from build123d import *

# Parameters (mm, degrees)
SKIZZE1_W                       = 660
SKIZZE1_H                       = 370
AUFSATZ_LINEAR_AUSTRAGEN1_DEPTH = 200
SKIZZE2_R                       = 30
SCHNITT_LINEAR_AUSTRAGEN1_DEPTH = 566.799856976
VERRUNDUNG1_R                   = 30
SKIZZE3_W                       = 300
SKIZZE3_H                       = 270
SCHNITT_LINEAR_AUSTRAGEN2_DEPTH = 30
VERRUNDUNG2_R                   = 30
SKIZZE5_W                       = 50
SKIZZE5_H                       = 100
AUFSATZ_LINEAR_AUSTRAGEN2_DEPTH = 200


with BuildPart() as part:
    # Skizze1 → Aufsatz-Linear austragen1 (new body)
    with BuildSketch(Plane.XY):
        with Locations((-48.456705786, -9.625748503)):
            Rectangle(SKIZZE1_W, SKIZZE1_H)
    extrude(amount=AUFSATZ_LINEAR_AUSTRAGEN1_DEPTH)

    # Skizze2 → Schnitt-Linear austragen1 (cut, through all)
    with BuildSketch(Plane.XZ.offset(194.625748503)):
        with Locations(Location((-303.456705786, 80, 0), (0, 0, 270))):
            Circle(SKIZZE2_R)
        with Locations(Location((206.543294214, 80, 0), (0, 0, 270))):
            Circle(SKIZZE2_R)
    extrude(amount=-SCHNITT_LINEAR_AUSTRAGEN1_DEPTH, mode=Mode.SUBTRACT)

    # Verrundung1
    verrundung1_edges = [part.edges().sort_by_distance(p)[0] for p in [
        (281.543294214, -9.625748503, 200),
        (-48.456705786, 175.374251497, 200),
        (-378.456705786, -9.625748503, 200),
        (281.543294214, -9.625748503, 0),
        (-378.456705786, -9.625748503, 0),
        (-378.456705786, 175.374251497, 100),
        (281.543294214, 175.374251497, 100),
        (281.543294214, -194.625748503, 100),
        (-378.456705786, -194.625748503, 100),
        (-48.456705786, -194.625748503, 200),
    ]]
    fillet(verrundung1_edges, radius=VERRUNDUNG1_R)

    # Skizze3 → Schnitt-Linear austragen2 (cut)
    with BuildSketch(Plane.XY.offset(200)):
        with Locations((83.717618878, -9.625748503)):
            Rectangle(SKIZZE3_W, SKIZZE3_H)
    extrude(amount=-SCHNITT_LINEAR_AUSTRAGEN2_DEPTH, mode=Mode.SUBTRACT)

    # Verrundung2
    verrundung2_edges = [part.edges().sort_by_distance(p)[0] for p in [
        (233.717618878, -9.625748503, 170),
        (83.717618878, -144.625748503, 170),
        (-66.282381122, -9.625748503, 170),
        (83.717618878, 125.374251497, 170),
    ]]
    fillet(verrundung2_edges, radius=VERRUNDUNG2_R - 0.0001)  # a hair under: the kernel refuses the full size

    # Skizze5 → Aufsatz-Linear austragen2 (add)
    with BuildSketch(Plane.XY.offset(200)):
        with Locations((-207.369543454, -9.625748503)):
            Rectangle(SKIZZE5_W, SKIZZE5_H)
    extrude(amount=AUFSATZ_LINEAR_AUSTRAGEN2_DEPTH)


solid = part.part
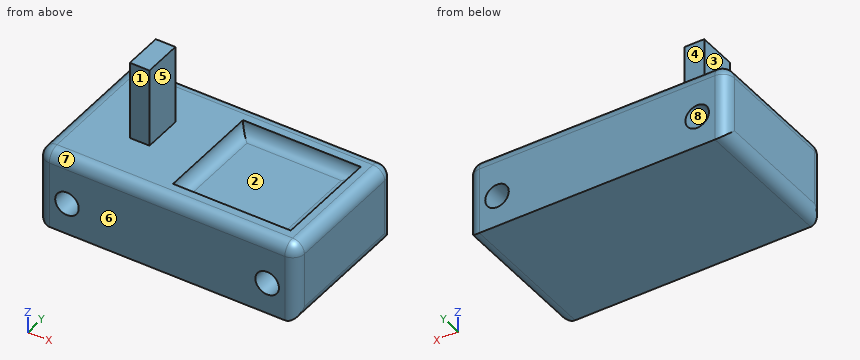
Work out the finished part from the listing and answer in its coordinate system (mm). Face numbers are marked on the shaded views. A direction names the side the tool comes from. Coordinates: 2 decimals unless noted, no trailing zeros. Loops run counter-clockwise (first coordinate to the right, second up) from the corner with the lowest first, then second, coordinate; pieces in that order, holes last. Notation, with made-up numbers: M 81.25,-5 L 128.25,-5 A17 cw 128.25,21 Z; hole C -20,-25 d7. An arc over 180 degrees is marked long. Answer in a Markdown table with one row per item. Add a question column.
1. Find section A-A, the plane z = 80. Write down the section's boundary in (x, y).
2. Find section D-D, the plane z = 188. Write down the section's boundary in (x, y).
3. A tool of negligible diameter and unlimited length cuts with its end or side. For the marked faces 1, 2, 3, 4 and 5, from which of +Z, -Z, +X, -X, +Y, -Y can it reach the whole face along a straight path? Write none if from no direction.
4. The mould has two halves that part along Z. Classify the marked faces 6, 7 and 8: pulls with the +Z half, pulls with the -Z half, needs draft (parallel to the pull), parting line crosses it, or undercut.
5. Consider L1, parallel to X at y = 100, z = 80; L2, parallel to Z at x = 203.5, y = -75; L3, parallel to X at y = 16, z = 59. Determine where each line is inside the solid, lowest interval first.
6. Find section C-C, the plane y = 103. State how many separate pieces and enclosed holes the cut face has, then the cut area to 3 significant figures.
7. Flat-ended cylindrical pins translate along their axes: P1, Ø3, axis at y = 31.5, z = 243, coming from the -X side; P2, Ø1, axis at x = 130, y = 76.5, coming from the +Z side; P3, Ø1.5, axis at x = -268, y = -83.5, coming from the +Z side; P4, Ø3, axis at y = -62.5, z = 339.5, coming from the -X side. Find the tip coordinate at first contact, or state that the pin passes through.
Reported:
| question | item | result |
|---|---|---|
| 1 | outline | M -378.46,-164.63 A30 ccw -348.46,-194.63 L -333.46,-194.63 L -333.46,175.37 L -348.46,175.37 A30 ccw -378.46,145.37 Z; M -273.46,-194.63 L 176.54,-194.63 L 176.54,175.37 L -273.46,175.37 Z; M 236.54,-194.63 L 251.54,-194.63 A30 ccw 281.54,-164.63 L 281.54,145.37 A30 ccw 251.54,175.37 L 236.54,175.37 Z |
| 2 | outline | M -372.46,-164.63 A24 ccw -348.46,-188.63 L 251.54,-188.63 A24 ccw 275.54,-164.63 L 275.54,145.37 A24 ccw 251.54,169.37 L -348.46,169.37 A24 ccw -372.46,145.37 Z; hole M -63.78,-142.12 L 231.21,-142.12 L 231.21,122.87 L -63.78,122.87 Z |
| 3 | face 1 | +Z, +X, -X, -Y |
| 3 | face 2 | +Z |
| 3 | face 3 | +Z, -X, +Y, -Y |
| 3 | face 4 | +Z, +X, -X, +Y |
| 3 | face 5 | +Z, +X, +Y, -Y |
| 4 | face 6 | needs draft |
| 4 | face 7 | pulls with the +Z half |
| 4 | face 8 | undercut |
| 5 | L1 | x = -378.46 to -333.46, -273.46 to 176.54, 236.54 to 281.54 |
| 5 | L2 | z = 0 to 50.15, 109.85 to 170 |
| 5 | L3 | x = -378.46 to -324.88, -282.03 to 185.12, 227.97 to 281.54 |
| 6 | separate pieces | 1 |
| 6 | enclosed holes | 2 |
| 6 | area | 117,000 mm^2 |
| 7 | P1 | stops at x = -232.37 |
| 7 | P2 | stops at z = 170 |
| 7 | P3 | stops at z = 200 |
| 7 | P4 | passes through |
